from build123d import *

# Parameters (mm, degrees)
BOSS_EXTRUDE1_DEPTH      = 0.1
BOSS_EXTRUDE1_DEPTH_BACK = 0.1
BOSS_EXTRUDE2_DEPTH      = 0.1
BOSS_EXTRUDE2_DEPTH_BACK = 0.1


with BuildPart() as part:
    # Sketch1 → Boss-Extrude1 (new, two sides: drawn at the far end of the back side and taken through both)
    with BuildSketch(Plane(origin=(0, 0, 0), x_dir=(1, 0, 0), z_dir=(0, 1, 0)).offset(-BOSS_EXTRUDE1_DEPTH_BACK)):
        Polygon((8, -3), (1, -2), (1, -5), (0, -7), (0, 5), (1, 4), (1, 1), (8, -2), align=None)
        Polygon((-1, 4), (-1, 1), (-8, -2), (-8, -3), (-1, -2), (-1, -5), (0, -7), (0, 5), align=None)
        Polygon((1, 1), (8, -2), (8, -3), (1, -2), align=None)
        Polygon((-8, -3), (-1, -2), (-1, 1), (-8, -2), align=None)
    extrude(amount=BOSS_EXTRUDE1_DEPTH + BOSS_EXTRUDE1_DEPTH_BACK)

    # Sketch2 → Boss-Extrude2 (add, two sides: drawn at the far end of the back side and taken through both)
    with BuildSketch(Plane(origin=(0, 0, 0), x_dir=(0, 0, -1), z_dir=(1, 0, 0)).offset(-BOSS_EXTRUDE2_DEPTH_BACK)):
        Polygon((5, 0), (4, 1), (-5, 1), (-6, 2), (-7, 2), (-7, 0), (-4, -1), (2, -1), align=None)
    extrude(amount=BOSS_EXTRUDE2_DEPTH + BOSS_EXTRUDE2_DEPTH_BACK)


solid = part.part
Work out the finished part from the listing and answer in its coordinate system (mm). A direction names the side the tool comes from. Give positions to 0.01 mm unless a question says otherwise; leave off trailing zeros. Write each loop counter-clockwise with the first axis right and the second up, starting at its lowest first coordinate (ties: lowest second). Pieces come first, ordered by that corner, then holes. Notation, with made-up numbers: M 35.25,10 L 67.25,10 A21 ccw 67.25,44 Z; hole C -10.5,-31 d7. An arc over 180 degrees is marked long. Answer as CSV lines item,"result".
Q1. Find the intervals of material crossed by probe 1 along X at (y, z) = (0.4, -3.5); probe 2 along Z at (x, y) = (0, 0.65), in increasing order. Write a range as [from, to].
A:
probe 1,"x = [-0.1, 0.1]"
probe 2,"z = [-4.35, 7]"
Q2. A tool of negligible diameter and unlimited length cuts with its end or side. For faces 1 (the flat face through (-3, 0.1, 1)), 2 (the flat face through (-0.1, -0.5, 1.1)), 3 (the flat face through (0.1, -0.5, 1.1)), 4 (the flat face through (3, 0.1, 1)), from which of +Z, -Z, +X, -X, +Y, -Y can it reach the whole face along a straight path? Write none if from no direction.
A:
face 1,"+Z, -Z, -X, +Y"
face 2,"+Z, -Z, -X, -Y"
face 3,"+Z, -Z, +X, -Y"
face 4,"+Z, -Z, +X, +Y"
Q3. A cutting plane is placed at A-A on z = 1.25. Write down the section's boundary in (x, y).
A:
outline,"M -6.25,-0.1 L -0.1,-0.1 L -0.1,-1 L 0.1,-1 L 0.1,-0.1 L 6.25,-0.1 L 6.25,0.1 L 0.1,0.1 L 0.1,1 L -0.1,1 L -0.1,0.1 L -6.25,0.1 Z"
Q4. A cutting plane is placed at D-D on x = 3.25. Write down the section's boundary in (y, z).
A:
outline,"M -0.1,-0.04 L 0.1,-0.04 L 0.1,2.32 L -0.1,2.32 Z"
Q5. A cutting plane is placed at B-B on y = 0.5. Write down the section's boundary in (x, z), plus the area to 3 significant figures.
A:
outline,"M -0.1,-4.5 L 0.1,-4.5 L 0.1,7 L -0.1,7 Z"
area,"2.30 mm²"
Q6. Given P1, Ø6.5, axis at x = 3.5, z = 0.5, coming from the +Y side; P2, Ø0.5, axis at y = -0.5, z = 3.5, coming from the -X side; P3, Ø5, axis at x = 1, z = -2.5, coming from the +Y side, each flat-ended and moving along its own axis, determine where each tip first touches the part or whether it passes through.
A:
P1,"stops at y = 0.1"
P2,"stops at x = -0.1"
P3,"stops at y = 1"
Q7. A cutting plane is placed at C-C on z = -1.5. Write down the section's boundary in (x, y).
A:
outline,"M -1,-0.1 L -0.1,-0.1 L -0.1,-1 L 0.1,-1 L 0.1,-0.1 L 1,-0.1 L 1,0.1 L 0.1,0.1 L 0.1,1 L -0.1,1 L -0.1,0.1 L -1,0.1 Z"
